Source: CAD feature listing. Evaluate the final solid. Frame: model axes, mm. A direction names the side the tool comes from. Round coordinates to 2 decimals unless told otherwise and drop trailing zeros. Order: outer loops, then holes, each group sorted by start corner. A loop starts at its lowest first (then second) coordinate and runs counter-clockwise, first axis right, second up. Notation, with made-up numbers: (34.25, -26.75) -> (76.25, -26.75) arc R25 ccw to (76.25, -0.75) -> close; hole circle Ø9 at (88, 18.25). An arc over 180 degrees is marked (long way). Answer as CSV lines item,"result". Start each with the question number.
(1) Contact query for flat-ended pins moving along their axis: P1, Ø3, axis at x = 68, y = -3, coming from the -Z side; P2, Ø4, axis at y = -13.5, z = 11.5, coming from the -X side; P3, Ø6, axis at x = 66, z = -0.5, coming from the +Y side. Output: stop coordinate, or through.
(2) Section query C-C (x = 9.75). Output: boundary loops of the cut face in (y, z).
(3) Set-up query: faces 1 (the flat face through (46.75, -36, -1)), 2 (the flat face through (15, -6, -2)), 3 (the cylindrical face through (26.2, -8.5, 6.6)). Return all of +Z, -Z, +X, -X, +Y, -Y with unobstructed straight access to the full face (end or side cutting, diameter ignored); none if empty.
(4) Section query D-D (x = 29.75). Output: boundary loops of the cut face in (y, z), plus the area to 3 significant figures.
(5) Line query: line 1 along Y through (x, z) = (97.8, 9.25); line 2 along X through (y, z) = (45.05, 1.5); line 3 along X through (y, z) = (-15, 3.75). Output: solid intervals per line, ascending. Write a range as from..to.
(6) Pull-direction query (Y, two-part tool) for faces 4 (the flat face through (38, 47.5, 7)), 5 (the flat face through (4.75, -11, -2)), 6 (the flat face through (48, 21, 0)); classes: +Y half, -Y half, draft (parallel to the pull), parting line (faces both ways), or undercut.
(7) Section query A-A (z = -1.5). Count the separate pieces of the cut face and the enclosed holes in it, plus the area to 3 significant figures.
```python
from build123d import *

# Parameters (mm, degrees)
EXTRUDE_1_DEPTH      = 16.5
SKETCH_2_R           = 2.5
CUT_EXTRUDE_1_DEPTH  = 16.5
SKETCH_3_W           = 10
SKETCH_3_H           = 16.5
CUT_EXTRUDE_2_DEPTH  = 3
SKETCH_4_W           = 11.896315449
SKETCH_4_H           = 29.084641161
CUT_EXTRUDE_3_DEPTH  = 48.945933091
SKETCH_5_R           = 2
CUT_EXTRUDE_4_DEPTH  = 48.945933091
SKETCH_6_W           = 10
SKETCH_6_H           = 23
EXTRUDE_2_DEPTH      = 3
SKETCH_7_R           = 2.5
CUT_EXTRUDE_5_DEPTH  = 3
EXTRUDE_START        = 3
SKETCH_8_R           = 2
SKETCH_8_W           = 6
SKETCH_8_H           = 26
EXTRUDE_3_DEPTH      = 3
SKETCH_9_R           = 2.5
CUT_EXTRUDE_6_DEPTH  = 3
SKETCH_10_W          = 74.694005649
SKETCH_10_H          = 52.095093629
CUT_EXTRUDE_7_DEPTH  = 116.604119736
SKETCH_11_W          = 16.482634167
SKETCH_11_H          = 25.810545036
CUT_EXTRUDE_8_DEPTH  = 10
SKETCH_13_R          = 2
EXTRUDE_4_DEPTH      = 19.5
SKETCH_14_W          = 6
SKETCH_14_H          = 41.5
CUT_EXTRUDE_9_DEPTH  = 3
SKETCH_15_W          = 23
SKETCH_15_H          = 10
SKETCH_15_R          = 2.5
EXTRUDE_5_DEPTH      = 3
SKETCH_16_W          = 3
SKETCH_16_H          = 10
EXTRUDE_6_DEPTH      = 16.5
SKETCH_17_R          = 2.5
CUT_EXTRUDE_10_DEPTH = 3


with BuildPart() as part:
    # 草图1 → 凸台-拉伸1 (new body)
    with BuildSketch(Plane.XY):
        Polygon((0, 0), (26.75, 0), (26.75, -20), (36.75, -20), (36.75, -26), (20.75, -26), (20.75, -6), (0, -6), (-20.75, -6), (-20.75, -26), (-36.75, -26), (-36.75, -20), (-26.75, -20), (-26.75, 0), align=None)
    extrude(amount=EXTRUDE_1_DEPTH)

    # 草图2 → 切除-拉伸1 (cut)
    with BuildSketch(Plane(origin=(0, -20, 0), x_dir=(1, 0, 0), z_dir=(0, 1, 0))):
        with Locations(Location((32.75, -8.25, 0), (0, 0, 270))):
            Circle(SKETCH_2_R)
    extrude(amount=-CUT_EXTRUDE_1_DEPTH, mode=Mode.SUBTRACT)

    # 草图3 → 切除-拉伸2 (cut)
    with BuildSketch(Plane(origin=(0, -20, 0), x_dir=(1, 0, 0), z_dir=(0, 1, 0))):
        with Locations((31.75, -8.25)):
            Rectangle(SKETCH_3_W, SKETCH_3_H)
    extrude(amount=-CUT_EXTRUDE_2_DEPTH, mode=Mode.SUBTRACT)

    # 草图4 → 切除-拉伸3 (cut, through all)
    with BuildSketch(Plane.XY.offset(16.5)):
        with Locations((-32.698157724, -14.542320581)):
            Rectangle(SKETCH_4_W, SKETCH_4_H)
    extrude(amount=-CUT_EXTRUDE_3_DEPTH, mode=Mode.SUBTRACT)

    # 草图5 → 切除-拉伸4 (cut, through all)
    with BuildSketch(Plane(origin=(0, 0, 0), x_dir=(-1, 0, 0), z_dir=(0, 0, -1))):
        with Locations((-24.3, -11)):
            Circle(SKETCH_5_R)
        with Locations((-24.3, -21)):
            Circle(SKETCH_5_R)
        with Locations(Location((24.3, -21, 0), (0, 0, 180))):
            Circle(SKETCH_5_R)
        with Locations(Location((24.3, -11, 0), (0, 0, 180))):
            Circle(SKETCH_5_R)
    extrude(amount=-CUT_EXTRUDE_4_DEPTH, mode=Mode.SUBTRACT)

    # 草图6 → 凸台-拉伸2 (add)
    with BuildSketch(Plane(origin=(0, 0, 0), x_dir=(-1, 0, 0), z_dir=(0, 0, -1))):
        with Locations((-31.75, -34.5)):
            Rectangle(SKETCH_6_W, SKETCH_6_H)
    extrude(amount=EXTRUDE_2_DEPTH)

    # 草图7 → 切除-拉伸5 (cut)
    with BuildSketch(Plane(origin=(0, 0, -3), x_dir=(-1, 0, 0), z_dir=(0, 0, -1))):
        with Locations((-31.75, -36)):
            Circle(SKETCH_7_R)
    extrude(amount=-CUT_EXTRUDE_5_DEPTH, mode=Mode.SUBTRACT)

    # 草图8 → 凸台-拉伸3 (add)
    # profile 1 of 2: a face of its own
    with BuildSketch(Plane(origin=(0, 0, 0), x_dir=(-1, 0, 0), z_dir=(0, 0, -1)).offset(EXTRUDE_START)):
        Polygon((26.75, 0), (20.75, 0), (20.75, -46), (26.75, -46), (30.75, -46), (30.75, -26), (26.75, -26), align=None)
        with Locations((24.3, -21)):
            Circle(SKETCH_8_R, mode=Mode.SUBTRACT)
        with Locations((24.3, -11)):
            Circle(SKETCH_8_R, mode=Mode.SUBTRACT)
    # profile 2 of 2: a face of its own
    with BuildSketch(Plane(origin=(0, 0, 0), x_dir=(-1, 0, 0), z_dir=(0, 0, -1)).offset(EXTRUDE_START)):
        with Locations((-23.75, -13)):
            Rectangle(SKETCH_8_W, SKETCH_8_H)
        with Locations((-24.3, -11)):
            Circle(SKETCH_8_R, mode=Mode.SUBTRACT)
        with Locations((-24.3, -21)):
            Circle(SKETCH_8_R, mode=Mode.SUBTRACT)
    extrude(amount=-EXTRUDE_3_DEPTH)

    # 草图9 → 切除-拉伸6 (cut)
    with BuildSketch(Plane(origin=(0, 0, -3), x_dir=(-1, 0, 0), z_dir=(0, 0, -1))):
        with Locations((25.75, -36)):
            Circle(SKETCH_9_R)
    extrude(amount=-CUT_EXTRUDE_6_DEPTH, mode=Mode.SUBTRACT)

    # 镜向1: part across plane


with BuildPart() as part_1:
    add(part.part)
    add(part.part.mirror(Plane(origin=(36.75, -20, 16.5), x_dir=(0, 0, 1), z_dir=(-1, 0, 0))))

    # 草图10 → 切除-拉伸7 (cut, through all)
    with BuildSketch(Plane(origin=(0, 0, -3), x_dir=(-1, 0, 0), z_dir=(0, 0, -1))):
        with Locations((0.597002825, -19.952453186)):
            Rectangle(SKETCH_10_W, SKETCH_10_H)
    extrude(amount=-CUT_EXTRUDE_7_DEPTH, mode=Mode.SUBTRACT)

    # 草图11 → 切除-拉伸8 (cut)
    with BuildSketch(Plane(origin=(0, 0, -3), x_dir=(-1, 0, 0), z_dir=(0, 0, -1))):
        with Locations((-102.491317084, -38.905272518)):
            Rectangle(SKETCH_11_W, SKETCH_11_H)
    extrude(amount=-CUT_EXTRUDE_8_DEPTH, mode=Mode.SUBTRACT)

    # 草图13 → 凸台-拉伸4 (add)
    with BuildSketch(Plane(origin=(0, 0, -3), x_dir=(-1, 0, 0), z_dir=(0, 0, -1))):
        Polygon((-24.75, -6), (-50.75, -6), (-50.75, 47.5), (-24.75, 47.5), (-24.75, 41.5), (-44.75, 41.5), (-44.75, 0), (-24.75, 0), align=None)
        with Locations((-29.75, -3.55)):
            Circle(SKETCH_13_R, mode=Mode.SUBTRACT)
        with Locations((-39.75, -3.55)):
            Circle(SKETCH_13_R, mode=Mode.SUBTRACT)
        with Locations(Location((-39.75, 45.05, 0), (0, 0, 180))):
            Circle(SKETCH_13_R, mode=Mode.SUBTRACT)
        with Locations(Location((-29.75, 45.05, 0), (0, 0, 180))):
            Circle(SKETCH_13_R, mode=Mode.SUBTRACT)
    extrude(amount=-EXTRUDE_4_DEPTH)

    # 草图14 → 切除-拉伸9 (cut)
    with BuildSketch(Plane(origin=(0, 0, -3), x_dir=(-1, 0, 0), z_dir=(0, 0, -1))):
        with Locations((-47.75, 20.75)):
            Rectangle(SKETCH_14_W, SKETCH_14_H)
    extrude(amount=-CUT_EXTRUDE_9_DEPTH, mode=Mode.SUBTRACT)

    # 草图15 → 凸台-拉伸5 (add)
    with BuildSketch(Plane(origin=(0, 0, -3), x_dir=(-1, 0, 0), z_dir=(0, 0, -1))):
        with Locations((-16.25, -11)):
            Rectangle(SKETCH_15_W, SKETCH_15_H)
        with Locations((-9.75, -11)):
            Circle(SKETCH_15_R, mode=Mode.SUBTRACT)
    extrude(amount=-EXTRUDE_5_DEPTH)

    # 草图16 → 凸台-拉伸6 (add)
    with BuildSketch(Plane.XY):
        with Locations((26.25, -11)):
            Rectangle(SKETCH_16_W, SKETCH_16_H)
    extrude(amount=EXTRUDE_6_DEPTH)

    # 草图17 → 切除-拉伸10 (cut)
    with BuildSketch(Plane.ZY.offset(-24.75)):
        with Locations(Location((6.5, -11, 0), (0, 0, 270))):
            Circle(SKETCH_17_R)
    extrude(amount=-CUT_EXTRUDE_10_DEPTH, mode=Mode.SUBTRACT)


solid = part_1.part
```
Answer block:
1,P1,"z = 0"
1,P2,"x = 24.75"
1,P3,"y = 0"
2,outline,"(-16, -3) -> (-13.5, -3) -> (-13.5, 0) -> (-16, 0) -> close; (-8.5, -3) -> (-6, -3) -> (-6, 0) -> (-8.5, 0) -> close"
3,face 1,"+Z, -Z, +X, -Y"
3,face 2,"+Z, -Z, -X, +Y"
3,face 3,"-X"
4,outline,"(-6, -3) -> (-5.55, -3) -> (-5.55, 16.5) -> (-6, 16.5) -> close; (-1.55, -3) -> (0, -3) -> (0, 16.5) -> (-1.55, 16.5) -> close; (41.5, -3) -> (43.05, -3) -> (43.05, 16.5) -> (41.5, 16.5) -> close; (47.05, -3) -> (47.5, -3) -> (47.5, 16.5) -> (47.05, 16.5) -> close"
4,area,"78.0 mm2"
5,line 1,"-26..-23, -19..-13, -9..0"
5,line 2,"24.75..27.75, 31.75..37.75, 41.75..50.75"
5,line 3,"24.75..27.75, 46.75..52.75, 94.25..100.25"
6,face 4,"+Y half"
6,face 5,"draft"
6,face 6,"undercut"
7,separate pieces,"3"
7,enclosed holes,"10"
7,area,"920 mm2"
